Part model, mm, in its own coordinate system. A direction names the side the tool comes from. Coordinates: 2 decimals unless noted, no trailing zeros. Loops run counter-clockwise (first coordinate to the right, second up) from the corner with the lowest first, then second, coordinate; pieces in that order, holes last. Notation, with made-up numbers: (64.25, 60.25) - (75.25, 60.25) arc R22 ccw to (75.25, 83.25) - close; hole circle Ø6 at (28, 68). An arc over 180 degrees is marked (long way). One line per question, with ' | ' between items. Start each with the question number.
Autodesk Fusion 360 part; units mm, degrees
sketch "Sketch1" plane through (0, 0, 0) normal (0, 0, 1) x (1, 0, 0)
  line L0 (0, 0) -> (-0.9251, 0)
  line L1 (-0.6, -0.8) -> (0, -0.8)
  line L2 (0, -0.8) -> (0, 0)
  line L3 (-0.6, -0.8) -> (-0.6, -1.6)
  line L4 (-0.6, -1.6) -> (0, -1.6)
  line L5 (0, -1.6) -> (0, -2.6)
  line L6 (-8.4, -2.6) -> (-8.4, -0.0952)
  line L7 (-16.8, -1.6) -> (-16.8, -2.6)
  line L8 (-16.2, -1.6) -> (-16.8, -1.6)
  line L9 (-16.2, -0.8) -> (-16.2, -1.6)
  line L10 (-16.2, -0.8) -> (-16.8, -0.8)
  line L11 (-16.8, -0.8) -> (-16.8, 0)
  line L12 (-16.8, -2.6) -> (-8.4, -2.6)
  line L13 (-16.8, 0) -> (0, 0)
  line L14 (0, -2.6) -> (-16.8, -2.6)
  dimension "d1" = 1
  dimension "d2" = 0.8
  dimension "d3" = 0.8
  dimension "d4" = 0.6
  dimension "d6" = 16.8
extrude "Extrude1" add sketch "Sketch1" along normal blind 14.5
sketch "Sketch2" plane through (0, 0, 0) normal (1, 0, 0) x (0, 1, 0)
  line L0 (-2.6, 0) -> (-1.6, 0)
  line L1 (-1.6, 0) -> (-1.6, 14.5)
  line L2 (-1.6, 14.5) -> (-2.6, 14.5)
  line L3 (-2.6, 14.5) -> (-2.6, 0)
  line L4 (-2.6, 0) -> (-2.6, 14.5)
  line L5 (-1.6, 0) -> (-2.6, 0)
  line L6 (-2.6, 0) -> (-4.6, 0)
  line L7 (-4.6, 0) -> (-2.6, 3.4641)
  line L8 (-4.1, 0) -> (-4.1, 0.866)
  point P0 (-2.6, 0)
  dimension "d9" = 60
  dimension "d10" = 2
  dimension "d17" = 1.5
extrude "Extrude2" add sketch "Sketch2" against normal blind 16.8 contours L3 L4 L6 L7 L8
sketch "Sketch3" plane through (0, 0, 0) normal (0, 1, 0) x (-1, 0, 0)
  line L0 (0, 0) -> (16.8, 0)
  line L1 (16.8, 0) -> (16.8, 14.5)
  line L2 (16.8, 14.5) -> (0, 14.5)
  line L3 (0, 14.5) -> (0, 0)
  line L4 (0, 14.5) -> (16.8, 14.5)
  line L5 (8.4, 14.5) -> (8.4, 8) construction
  line L6 (1.9, 14.5) -> (1.9, 8)
  line L7 (14.9, 14.5) -> (14.9, 8)
  arc A0 (1.9, 8) -> (14.9, 8) centre (8.4, 8) ccw
  dimension "d13" = 6.5
  dimension "d14" = 13
extrude "Extrude3" cut sketch "Sketch3" against normal blind 1 contours L2 L4 L6 L7 A0
chamfer "Chamfer1" distance 0.4 angle 45 4 edges at (-16.5, -0.8, 14.5) (-16.5, -1.6, 14.5) (-0.3, -0.8, 14.5) (-0.3, -1.6, 14.5)
sketch "Sketch4" plane through (0, 0, 0) normal (0, 1, 0) x (-1, 0, 0)
  line L0 (1.9, 8) -> (1.9, 14.5)
  line L1 (1.9, 14.5) -> (0, 14.5)
  line L2 (0, 14.5) -> (0, 0)
  line L3 (0, 0) -> (16.8, 0)
  line L4 (16.8, 0) -> (16.8, 14.5)
  line L5 (16.8, 14.5) -> (14.9, 14.5)
  line L6 (14.9, 14.5) -> (14.9, 8)
  arc A0 (1.9, 8) -> (14.9, 8) centre (8.4, 8) ccw
  line L7 (1.9, 14.5) -> (1.9, 0)
  line L8 (1.1, 0) -> (1.1, 14.5)
  dimension "d19" = 0.8
extrude "Extrude4" add sketch "Sketch4" along normal blind 10 contours L0 L1 L3 L7 L8
chamfer "Chamfer2" distance 10 angle 45 1 edges at (-1.5, 10, 14.5)
1) Wall check: line 1 along X through (y, z) = (5, 6.5); line 2 along Y through (x, z) = (-9.25, 7.5); line 3 along X through (y, z) = (-1.5, 3.5). Give the ranges that are in metal, low to high. Write a range as [from, to].
2) Pin check, flat tips, straight feed: pin 1 Ø0.5 at (x, z) = (-16.5, 9.5) entering from -Y; pin 2 Ø4 at (x, z) = (-11.5, 10) entering from +Y; pin 3 Ø0.5 at (x, z) = (-0.5, 5) entering from +Y. Stop position of each tip, or through.
3) Band-saw the part on C-C on y = 2. List the corners of the cut face in (x, z).
4) Band-saw the part on D-D on z = 7.25. List the corners of the cut face in (x, y), then the cut area to 3 significant figures.
5) Tool access for faces 5 (the flat face through (-1.5, 4.9, 9.6)), 6 (the flat face through (-13, 0, 3)), 7 (the flat face through (-8, -1, 8)), 8 (the flat face through (-0.5, 0, 7.1)), 9 (the flat face through (-8, -2.6, 9)): list every direction of +Z, -Z, +X, -X, +Y, -Y with a clear straight run to the whole face (end or side of a thin tool).
6) Band-saw the part on B-B on z = 9. List the corners of the cut face in (x, y), then the cut area to 3 significant figures.
7) Band-saw the part on A-A on x = -8.4. List the corners of the cut face in (y, z).
8) Mould opens along X. For faces 1 (the flat face through (-8.28, -3.36, 2.15)), 2 (the flat face through (-1.1, 4, 6)), 3 (the flat face through (-14.9, -0.5, 11.3)), 4 (the flat face through (-16.2, -1, 7)) say: +X half, -X half, draft (parallel to the pull), parting line (faces both ways), or undercut.
Values found:
1) line 1: [-1.9, -1.1] | line 2: [-2.6, -1] | line 3: [-16.2, -0.6]
2) pin 1: y = -2.6 | pin 2: y = -1 | pin 3: y = 0
3) outline: (-1.9, 0) - (-1.1, 0) - (-1.1, 12.5) - (-1.9, 12.5) - close
4) outline: (-16.8, -2.6) - (0, -2.6) - (0, -1.6) - (-0.6, -1.6) - (-0.6, -0.8) - (0, -0.8) - (0, 0) - (-1.1, 0) - (-1.1, 7.25) - (-1.9, 7.25) - (-1.9, 0) - (-1.94, 0) - (-1.94, -1) - (-14.86, -1) - (-14.86, 0) - (-16.8, 0) - (-16.8, -0.8) - (-16.2, -0.8) - (-16.2, -1.6) - (-16.8, -1.6) - close | area: 35.6 mm²
5) face 5: +Z, +X, -X, +Y | face 6: +Z, -Z, -X, +Y | face 7: +Z, +Y | face 8: +Z, -Z, +X, +Y | face 9: +Z, +X, -X, -Y
6) outline: (-16.8, -2.6) - (0, -2.6) - (0, -1.6) - (-0.6, -1.6) - (-0.6, -0.8) - (0, -0.8) - (0, 0) - (-1.1, 0) - (-1.1, 5.5) - (-1.9, 5.5) - (-1.9, -1) - (-14.9, -1) - (-14.9, 0) - (-16.8, 0) - (-16.8, -0.8) - (-16.2, -0.8) - (-16.2, -1.6) - (-16.8, -1.6) - close | area: 34.1 mm²
7) outline: (-4.1, 0) - (0, 0) - (0, 1.5) - (-1, 1.5) - (-1, 14.5) - (-2.6, 14.5) - (-2.6, 3.46) - (-4.1, 0.87) - close
8) face 1: draft | face 2: +X half | face 3: undercut | face 4: -X half
